Read the model definition and answer for the solid it produces. Units are mm, in the model's axes. Coordinates: 2 decimals unless noted, no trailing zeros. Loops run counter-clockwise (first coordinate to the right, second up) from the corner with the lowest first, then second, coordinate; pieces in that order, holes last.
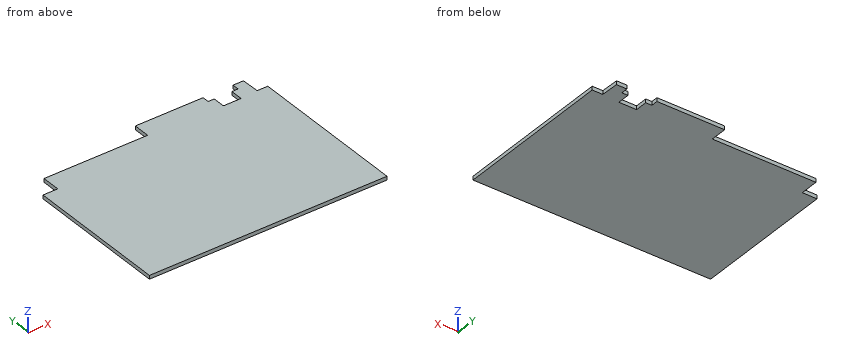
from build123d import *

# Parameters (mm, degrees)
BOSS_EXTRUDE1_DEPTH = 6
SKETCH2_W           = 30
SKETCH2_H           = 30
CUT_EXTRUDE1_DEPTH  = 10
SKETCH3_W           = 398.694966145
SKETCH3_H           = 1
CUT_EXTRUDE2_DEPTH  = 10
SKETCH4_W           = 6
SKETCH4_H           = 233
SKETCH4_H_2         = 258.947078575
CUT_EXTRUDE3_DEPTH  = 10
SKETCH5_W           = 23
SKETCH5_H           = 31.052921425
CUT_EXTRUDE4_DEPTH  = 10
SKETCH6_W           = 10
SKETCH6_H           = 20
BOSS_EXTRUDE2_DEPTH = 6
SKETCH7_W           = 17.21166374
SKETCH7_H           = 2.05
BOSS_EXTRUDE3_DEPTH = 6


with BuildPart() as part:
    # Sketch1 → Boss-Extrude1 (new body)
    with BuildSketch(Plane.XY):
        Polygon((28.571428571, 236.060202245), (28.571428571, 237.05184048), (5.415486436, 237.05184048), (4.571428571, 268.104761905), (-12.428571429, 268.104761905), (-12.428571429, 237.05184048), (-38.216595912, 237.05184048), (-38.216595912, 268.104761905), (-171.428571429, 268.104761905), (-171.428571429, 241.104761905), (-370.123537574, 241.104761905), (-370.123537574, -22.895238095), (28.571428571, -22.895238095), align=None)
    extrude(amount=BOSS_EXTRUDE1_DEPTH)

    # Sketch2 → Cut-Extrude1 (cut)
    with BuildSketch(Plane.XY.offset(6)):
        with Locations((-355.123537574, 226.104761905)):
            Rectangle(SKETCH2_W, SKETCH2_H)
    extrude(amount=-CUT_EXTRUDE1_DEPTH, mode=Mode.SUBTRACT)

    # Sketch3 → Cut-Extrude2 (cut)
    with BuildSketch(Plane.XY.offset(6)):
        with Locations((-170.776054501, -22.395238095)):
            Rectangle(SKETCH3_W, SKETCH3_H)
    extrude(amount=-CUT_EXTRUDE2_DEPTH, mode=Mode.SUBTRACT)

    # Sketch4 → Cut-Extrude3 (cut)
    with BuildSketch(Plane.XY.offset(6)):
        with Locations((-367.123537574, 94.604761905)):
            Rectangle(SKETCH4_W, SKETCH4_H)
        with Locations((25.571428571, 107.578301193)):
            Rectangle(SKETCH4_W, SKETCH4_H_2)
    extrude(amount=-CUT_EXTRUDE3_DEPTH, mode=Mode.SUBTRACT)

    # Sketch5 → Cut-Extrude4 (cut)
    with BuildSketch(Plane.XY.offset(6)):
        with Locations((-49.716595912, 252.578301193)):
            Rectangle(SKETCH5_W, SKETCH5_H)
    extrude(amount=-CUT_EXTRUDE4_DEPTH, mode=Mode.SUBTRACT)

    # Sketch6 → Boss-Extrude2 (add)
    with BuildSketch(Plane.XY.offset(6)):
        with Locations((-17.428571429, 247.05184048)):
            Rectangle(SKETCH6_W, SKETCH6_H)
        with Locations((-56.216595912, 247.05184048)):
            Rectangle(SKETCH6_W, SKETCH6_H)
    extrude(amount=-BOSS_EXTRUDE2_DEPTH)

    # Sketch7 → Boss-Extrude3 (add)
    with BuildSketch(Plane.XY.offset(6)):
        with Locations((13.965596701, 238.07684048)):
            Rectangle(SKETCH7_W, SKETCH7_H)
    extrude(amount=-BOSS_EXTRUDE3_DEPTH)


solid = part.part
Item 1: A cutting plane is placed at C-C on x = -276. Determine the outline of the cut face in (y, z), then the cut area to 3 significant figures.
Numbers:
outline: (-21.9, 0) - (241.1, 0) - (241.1, 6) - (-21.9, 6) - close
area: 1,580 mm2
Item 2: Find the intervals of material crossed by line 1 along Y through (x, z) = (-58, 4.05); line 2 along Y through (x, z) = (-36, 0.7); line 3 along X through (y, z) = (216, 3.55), in increasing order.
Numbers:
line 1: y = -21.9 to 257.05
line 2: y = -21.9 to 237.05
line 3: x = -340.12 to 22.57
Item 3: A cutting plane is placed at B-B on y = 246. Determine the outline of the cut face in (x, z).
Numbers:
outline: (-171.43, 0) - (-51.22, 0) - (-51.22, 6) - (-171.43, 6) - close; (-22.43, 0) - (5.17, 0) - (5.17, 6) - (-22.43, 6) - close
Item 4: A cutting plane is placed at A-A on z = 2.95. Determine the outline of the cut face in (x, y).
Numbers:
outline: (-364.12, -21.9) - (22.57, -21.9) - (22.57, 239.1) - (5.36, 239.1) - (4.57, 268.1) - (-12.43, 268.1) - (-12.43, 257.05) - (-22.43, 257.05) - (-22.43, 237.05) - (-51.22, 237.05) - (-51.22, 257.05) - (-61.22, 257.05) - (-61.22, 268.1) - (-171.43, 268.1) - (-171.43, 241.1) - (-340.12, 241.1) - (-340.12, 211.1) - (-364.12, 211.1) - close
Item 5: Given pin 1 (2 mm diameter, centred on x = -186, z = 4.5, fed in from +Y); pin 2 (3 mm diameter, centred on x = -31, z = 4, fed in from +Y); pin 3 (3 mm diameter, centred on x = -54, z = 3.5, fed in from +Y), each flat-ended and moving along its own axis, determine where each tip first touches the part or whether it passes through.
Numbers:
pin 1: stops at y = 241.1
pin 2: stops at y = 237.05
pin 3: stops at y = 257.05
